from build123d import *

# Parameters (mm, degrees)
F0_R     = 9.4996
F1_DEPTH = 5.461
F2_R     = 2.9845
F3_DEPTH = 12.0396
F4_R     = 2.8321
F5_DEPTH = 3.3782
F6_R     = 1.9939
F7_DEPTH = 4.445
F8_R     = 1.6002
F9_DEPTH = 25.4


with BuildPart() as f1:
    # F0 (on Top) → F1 (new body)
    with BuildSketch(Plane.XY):
        Circle(F0_R)
    extrude(amount=F1_DEPTH)

    # F2 (on face) → F3 (join)
    with BuildSketch(Plane.XY.offset(5.461)):
        Circle(F2_R)
    extrude(amount=F3_DEPTH)

    # F4 (on face) → F5 (cut)
    with BuildSketch(Plane.XY.offset(5.461)):
        with Locations((-5.8801, 0)):
            Circle(F4_R)
        with Locations((5.8801, 0)):
            Circle(F4_R)
    extrude(amount=-F5_DEPTH, mode=Mode.SUBTRACT)

    # F6 (on face) → F7 (cut)
    with BuildSketch(Plane(origin=(0, 0, 0), x_dir=(1, 0, 0), z_dir=(0, 0, -1))):
        Circle(F6_R)
    extrude(amount=-F7_DEPTH, mode=Mode.SUBTRACT)

    # F8 (on face) → F9 (cut)
    with BuildSketch(Plane(origin=(0, 0, 0), x_dir=(1, 0, 0), z_dir=(0, 0, -1))):
        with Locations((5.969, 0)):
            Circle(F8_R)
        with Locations((-5.969, 0)):
            Circle(F8_R)
    extrude(amount=-F9_DEPTH, mode=Mode.SUBTRACT)


solid = f1.part
For this review, take the finished solid that the model builds, in its own axes (mm). A direction names the side the tool comes from. Round coordinates to 2 decimals unless told otherwise and drop trailing zeros. Write each loop counter-clockwise with the first axis right and the second up, starting at its lowest first coordinate (ties: lowest second). Pieces come first, ordered by that corner, then holes. Notation, with made-up numbers: (86, 63.25) -> (95, 63.25) arc R26 ccw to (95, 87.25) -> close; hole circle Ø11 at (80, 64). An arc over 180 degrees is marked (long way). Put each result on its own line as item: value.
Q1. Machinability: for faces 4 (the cylindrical face through (1.9, -0.6, 2.2)), 5 (the flat face through (8, 0, 2.083)), 6 (the cylindrical face through (7.495, -0.481, 1.027)), which of the approach directions +Z, -Z, +X, -X, +Y, -Y give a long, thin tool a straight path to every point of the face, cutting with its end or side? Answer none if there is none.
Determined:
face 4: -Z
face 5: +Z
face 6: +Z, -Z
Q2. Clearance check with flat-ended pins moving along their axes: pin 1 Ø8 at (x, z) = (-6.5, 6.5) entering from -Y; pin 2 Ø6 at (x, y) = (-6, -1) entering from +Z; pin 3 Ø6 at (x, z) = (-6.5, 11.5) entering from +Y; pin 4 Ø3 at (x, z) = (-3, 12) entering from -Y. State where each tip first meets the part, or that it passes through.
Determined:
pin 1: stops at y = -9.13
pin 2: stops at z = 5.46
pin 3: passes through
pin 4: stops at y = -2.58
Q3. Consider section A-A on y = 0. Give the number of separate pieces and of enclosed holes in the cut face, and give its area (3 significant figures).
Determined:
separate pieces: 3
enclosed holes: 0
area: 106 mm^2
Q4. To check wall thickness, follow L1, parallel to Y at x = 0, z = 2.4; L2, parallel to Z at x = -1.5, y = 7; L3, parallel to Z at x = -7.25, y = -1. State the ranges of each line that lie inside material, in increasing order. Write a range as [from, to].
Determined:
L1: y = [-9.5, -1.99], [1.99, 9.5]
L2: z = [0, 5.46]
L3: z = [0, 2.08]
Q5. Consider section C-C on z = 1.25. State the section outline as (x, y) points, and give its area (3 significant figures).
Determined:
outline: circle Ø19 at (0, 0); hole circle Ø3.2 at (-5.97, 0); hole circle Ø3.99 at (0, 0); hole circle Ø3.2 at (5.97, 0)
area: 255 mm^2
Q6. Consider section B-B on x = 0. State the section outline as (y, z) points (1 decimal).
Determined:
outline: (-9.5, 0) -> (-2, 0) -> (-2, 4.4) -> (2, 4.4) -> (2, 0) -> (9.5, 0) -> (9.5, 5.5) -> (3, 5.5) -> (3, 17.5) -> (-3, 17.5) -> (-3, 5.5) -> (-9.5, 5.5) -> close
Q7. The part is to be moulded in two halves that separate along X. For faces 1 (the cylindrical face through (-7, 6.42, 2.69)), 2 (the flat face through (0, 0, 17.501)), 3 (the flat face through (0, 0, 4.445)), say which applies: released by +X, released by -X, zero draft, split by the parting line, or undercut.
Determined:
face 1: split by the parting line
face 2: zero draft
face 3: undercut
Q8. Consider section D-D on x = -6.5. State the section outline as (y, z) points, and give its area (3 significant figures).
Determined:
outline: (-6.93, 0) -> (-1.51, 0) -> (-1.51, 2.08) -> (-2.76, 2.08) -> (-2.76, 5.46) -> (-6.93, 5.46) -> close; (1.51, 0) -> (6.93, 0) -> (6.93, 5.46) -> (2.76, 5.46) -> (2.76, 2.08) -> (1.51, 2.08) -> close
area: 50.7 mm^2
